Can you work these out from the drawing? Everything is in mm from the part's minimum corner. A direction names the side the tool comes from. Give positions to 0.01 mm unless a question says otherwise; leave off trailing zeros. Write each loop counter-clockwise with the first axis right and the second up, starting at its lowest first coordinate (ties: lowest second). Pieces come first, ordered by that corner, then holes. Notation, with made-up numbers: M 81.5,-12 L 122.5,-12 A26 ccw 122.5,23 Z; hole C -30.5,64 d3. An arc over 180 degrees is marked long. One line per item, written item: value.
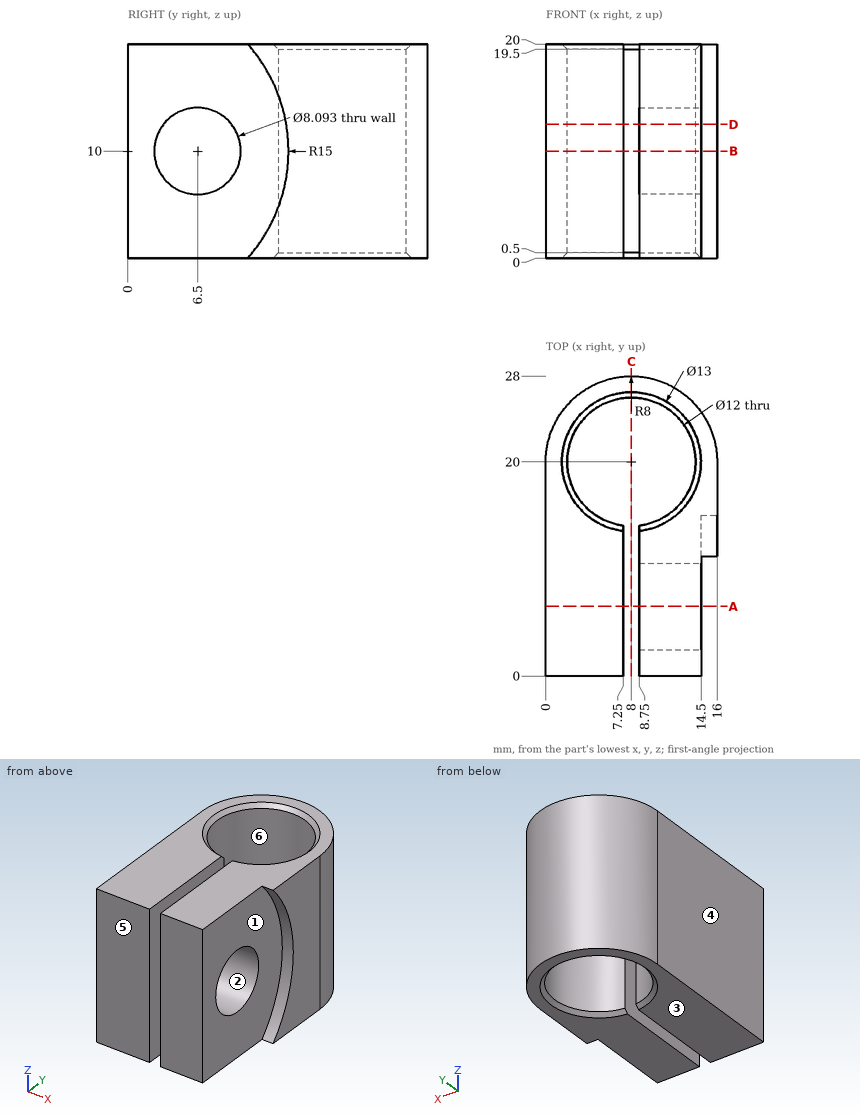
1) Please list where these lines run through material, in increasing order: L1, parallel to X at y = 12, z = 3.5; L2, parallel to X at y = 20, z = 13.75; L3, parallel to Y at x = 11.25, z = 10. Write a range as from..to.
Outcome:
L1: x = 0..7.25, 8.75..14.5
L2: x = 0..2, 14..16
L3: y = 0..2.45, 10.55..14.96, 25.04..27.31
2) If we section it at D-D, the plane z = 12.5: Write out the boundary of the cut face in (x, y), then the cut area to 3 significant figures.
Outcome:
outline: M 0,0 L 7.25,0 L 7.25,14.05 A6 cw long 8.75,14.05 L 8.75,9.68 L 14.5,9.68 L 14.5,14.79 L 16,14.79 L 16,20 A8 ccw 0,20 Z; M 8.75,0 L 14.5,0 L 14.5,3.32 L 8.75,3.32 Z
area: 228 mm^2
3) If we section it at C-C, the plane x = 8: Write out the boundary of the cut face in (y, z).
Outcome:
outline: M 26,0.5 L 26.5,0 L 28,0 L 28,20 L 26.5,20 L 26,19.5 Z
4) On a 3-axis mill with a long thin cutter (end or side, diameter ignored), from which of +Z, -Z, +X, -X, +Y, -Y can I reach the whole of each face in a straight line? I mean the marked faces 1, 2 and 3. Say none if no direction works.
Outcome:
face 1: +X, -Y
face 2: +X
face 3: -Z, +X, -X, +Y, -Y
5) If we section it at B-B, the plane z = 10: Write out the boundary of the cut face in (x, y), then the cut area to 3 significant figures.
Outcome:
outline: M 0,0 L 7.25,0 L 7.25,14.05 A6 cw long 8.75,14.05 L 8.75,10.55 L 14.5,10.55 L 14.5,15 L 16,15 L 16,20 A8 ccw 0,20 Z; M 8.75,0 L 14.5,0 L 14.5,2.45 L 8.75,2.45 Z
area: 217 mm^2
6) I'm going to push flat-ended pins straight in: pin 1 (4 mm diameter, centred on y = 24.5, z = 8.5, fed in from -X); pin 2 (3 mm diameter, centred on x = 13, z = 4, fed in from +Y); pin 3 (1 mm diameter, centred on x = 10.5, y = 24, fed in from -Z). Where does each tip first touch, or does it pass through?
Outcome:
pin 1: stops at x = 0.4
pin 2: stops at y = 27.19
pin 3: passes through
7) If we section it at A-A, the plane y = 6.5: Write out the boundary of the cut face in (x, z).
Outcome:
outline: M 0,0 L 7.25,0 L 7.25,20 L 0,20 Z; M 8.75,0 L 14.5,0 L 14.5,5.95 L 8.75,5.95 Z; M 8.75,14.05 L 14.5,14.05 L 14.5,20 L 8.75,20 Z
8) We'd pull the mould along Y, two halves only. Please class the marked faces 4, 5 and 6: pulls with the +Y half, pulls with the -Y half, needs draft (parallel to the pull), parting line crosses it, or undercut.
Outcome:
face 4: needs draft
face 5: pulls with the -Y half
face 6: undercut
